Geometry: final body of the model. Coordinates: model frame, mm. Give positions to 0.01 mm unless a question says otherwise; leave off trailing zeros. Order: outer loops, then holes, each group sorted by start corner. A loop starts at its lowest first (then second) coordinate and runs counter-clockwise, first axis right, second up. Notation, with made-up numbers: (-9.75, 1) -> (31.25, 1) arc R9 ccw to (31.25, 13) -> close; hole circle Ø3 at (-37.5, -15.75). An arc over 180 degrees is marked (long way). Write item = value, one per line.
```python
from build123d import *

# Parameters (mm, degrees)
F0_R            = 60
F0_R_2          = 30
F1_DEPTH        = 10
F3_D            = 11
F3_COPIES_COUNT = 6


# Not quite as in the source:
# - a pattern or mirror of a feature is missing from the dataset's text; its kind, count and spacing are read off the source's solid


with BuildPart() as f1:
    # F0 (on Top) → F1 (new body)
    with BuildSketch(Plane.XY):
        Circle(F0_R)
        Circle(F0_R_2, mode=Mode.SUBTRACT)
    extrude(amount=F1_DEPTH)

    # F3 (through all)
    with Locations(Plane.XY.offset(10)):
        with Locations((-50, 0)):
            f3 = Hole(F3_D / 2)

    # F3_copies: F3 ×6 about axis
    f3_copies_axis = Axis((0, 0, 0), (0, 0, 1))
    for i in range(1, F3_COPIES_COUNT):
        add(f3.rotate(f3_copies_axis, i * 360 / F3_COPIES_COUNT), mode=Mode.SUBTRACT)


solid = f1.part
```
1) Line query: line 1 (Y direction, x = -25, z = 5); line 2 (X direction, y = -38.5, z = 6.5); line 3 (Y direction, x = -25.5, z = 0.5). Output: solid intervals per line, ascending. Write a range as from..to.
Check sheet entries:
line_1 = -54.54..-48.8, -37.8..-16.58, 16.58..37.8, 48.8..54.54
line_2 = -46.02..-27.68, -22.32..22.32, 27.68..46.02
line_3 = -54.31..-48.78, -37.82..-15.8, 15.8..37.82, 48.78..54.31
2) Section query B-B (x = -25). Output: boundary loops of the cut face in (y, z).
Check sheet entries:
outline = (-54.54, 0) -> (-48.8, 0) -> (-48.8, 10) -> (-54.54, 10) -> close; (-37.8, 0) -> (-16.58, 0) -> (-16.58, 10) -> (-37.8, 10) -> close; (16.58, 0) -> (37.8, 0) -> (37.8, 10) -> (16.58, 10) -> close; (48.8, 0) -> (54.54, 0) -> (54.54, 10) -> (48.8, 10) -> close
3) Section query C-C (z = 6.75). Output: boundary loops of the cut face in (x, y), plus the area to 3 significant figures.
Check sheet entries:
outline = circle Ø120 at (0, 0); hole circle Ø11 at (-50, 0); hole circle Ø11 at (-25, -43.3); hole circle Ø11 at (-25, 43.3); hole circle Ø60 at (0, 0); hole circle Ø11 at (25, -43.3); hole circle Ø11 at (25, 43.3); hole circle Ø11 at (50, 0)
area = 7,910 mm²
4) Section query D-D (x = -9). Output: boundary loops of the cut face in (y, z), plus the area to 3 significant figures.
Check sheet entries:
outline = (-59.32, 0) -> (-28.62, 0) -> (-28.62, 10) -> (-59.32, 10) -> close; (28.62, 0) -> (59.32, 0) -> (59.32, 10) -> (28.62, 10) -> close
area = 614 mm²
5) Mould query, pull axis X, two halves, no side actions, for faces 1 (the face through (-29.05, -47.02, 4.93)), 2 (the face through (-59.94, 2.64, 4.93)), 3 (the face through (12, 28, 10)). Classes: +X half, -X half, draft (parallel to the pull), parting line (faces both ways), or undercut.
Check sheet entries:
face_1 = undercut
face_2 = parting line
face_3 = draft
6) Section query A-A (y = 44). Output: boundary loops of the cut face in (x, z).
Check sheet entries:
outline = (-40.79, 0) -> (-30.46, 0) -> (-30.46, 10) -> (-40.79, 10) -> close; (-19.54, 0) -> (19.54, 0) -> (19.54, 10) -> (-19.54, 10) -> close; (30.46, 0) -> (40.79, 0) -> (40.79, 10) -> (30.46, 10) -> close
7) First-contact query: P1, Ø1, axis at x = 11.5, z = 5, coming from the +Y side; P2, Ø12.5, axis at x = 25, y = -43.3, coming from the +Z side; P3, Ø5, axis at y = -42, z = 6.5, coming from the -X side; P4, Ø4, axis at y = 28.5, z = 4, coming from the -X side. Flat tips, straight axial feed; report the tip coordinate or a pass-through.
Check sheet entries:
P1 = 58.98
P2 = 10
P3 = -45.16
P4 = -53.83
